Source: CAD feature listing. Evaluate the final solid. Frame: model axes, mm. A direction names the side the tool comes from. Give positions to 0.01 mm unless a question says otherwise; leave off trailing zeros. Write each loop counter-clockwise with the first axis right and the second up, starting at its lowest first coordinate (ties: lowest second). Pieces come first, ordered by that corner, then holes. Notation, with made-up numbers: (-35, -30) -> (-8, -30) arc R11 ccw to (-8, -19) -> close; hole circle Ø7 at (-35.5, -18.5). An arc over 180 degrees is marked (long way). Write item = value, one per line.
from build123d import *

# Parameters (mm, degrees)
CROQUIS1_W                   = 60
CROQUIS1_H                   = 60
CROQUIS1_W_2                 = 48
CROQUIS1_H_2                 = 48
SALIENTE_EXTRUIR1_DEPTH      = 17.5
SALIENTE_EXTRUIR1_DEPTH_BACK = 17.5
CROQUIS2_R                   = 9
SALIENTE_EXTRUIR2_DEPTH      = 2
CROQUIS3_R                   = 9
SALIENTE_EXTRUIR3_DEPTH      = 2
CROQUIS4_R                   = 9
SALIENTE_EXTRUIR4_DEPTH      = 2
CROQUIS5_R                   = 5
SALIENTE_EXTRUIR5_DEPTH      = 63
SALIENTE_EXTRUIR5_DEPTH_BACK = 63
CROQUIS6_R                   = 5
SALIENTE_EXTRUIR6_DEPTH      = 68
CUT_EXTRUDE1_REACH           = 62
SKETCH1_R                    = 1.6


with BuildPart() as part:
    # Croquis1 → Saliente-Extruir1 (new body, two sides)
    with BuildSketch(Plane(origin=(0, 0, 0), x_dir=(1, 0, 0), z_dir=(0, 1, 0))) as saliente_extruir1_sk:
        Rectangle(CROQUIS1_W, CROQUIS1_H)
        Rectangle(CROQUIS1_W_2, CROQUIS1_H_2, mode=Mode.SUBTRACT)
    extrude(amount=SALIENTE_EXTRUIR1_DEPTH)
    extrude(saliente_extruir1_sk.sketch, amount=-SALIENTE_EXTRUIR1_DEPTH_BACK)

    # Croquis2 → Saliente-Extruir2 (add)
    with BuildSketch(Plane.XY.offset(30)):
        Circle(CROQUIS2_R)
    extrude(amount=SALIENTE_EXTRUIR2_DEPTH)

    # Croquis3 → Saliente-Extruir3 (add)
    with BuildSketch(Plane(origin=(30, 0, 0), x_dir=(0, 0, -1), z_dir=(1, 0, 0))):
        Circle(CROQUIS3_R)
    extrude(amount=SALIENTE_EXTRUIR3_DEPTH)

    # Croquis4 → Saliente-Extruir4 (add)
    with BuildSketch(Plane.ZY.offset(30)):
        Circle(CROQUIS4_R)
    extrude(amount=SALIENTE_EXTRUIR4_DEPTH)

    # Croquis5 → Saliente-Extruir5 (add, two sides)
    with BuildSketch(Plane(origin=(0, 0, 0), x_dir=(0, 0, -1), z_dir=(1, 0, 0))) as saliente_extruir5_sk:
        Circle(CROQUIS5_R)
    extrude(amount=SALIENTE_EXTRUIR5_DEPTH)
    extrude(saliente_extruir5_sk.sketch, amount=-SALIENTE_EXTRUIR5_DEPTH_BACK)

    # Croquis6 → Saliente-Extruir6 (add)
    with BuildSketch(Plane.XY):
        Circle(CROQUIS6_R)
    extrude(amount=SALIENTE_EXTRUIR6_DEPTH)

    # Sketch1 → Cut-Extrude1 (cut, up to next)
    with BuildSketch(Plane.XY.offset(30), mode=Mode.PRIVATE) as cut_extrude1_sk1:
        with Locations((-20, 0)):
            Circle(SKETCH1_R)
    cut_extrude1_tool1 = extrude(cut_extrude1_sk1.sketch, amount=-CUT_EXTRUDE1_REACH, mode=Mode.PRIVATE) & part.part
    add(cut_extrude1_tool1.solids().sort_by_distance((-20, 0, 30))[0], mode=Mode.SUBTRACT)
    # Sketch1 → Cut-Extrude1 (cut, up to next)
    with BuildSketch(Plane.XY.offset(30), mode=Mode.PRIVATE) as cut_extrude1_sk2:
        with Locations((20, 0)):
            Circle(SKETCH1_R)
    cut_extrude1_tool2 = extrude(cut_extrude1_sk2.sketch, amount=-CUT_EXTRUDE1_REACH, mode=Mode.PRIVATE) & part.part
    add(cut_extrude1_tool2.solids().sort_by_distance((20, 0, 30))[0], mode=Mode.SUBTRACT)


solid = part.part
1) Material intervals for L1, parallel to Y at x = -20, z = 26.05; L2, parallel to Z at x = -9, y = -9; L3, parallel to Z at x = 6, y = -6, sorted ascending.
Computed:
L1 = -17.5 to -1.6, 1.6 to 17.5
L2 = -30 to -24, 24 to 30
L3 = -30 to -24, 24 to 32
2) Contact query for flat-ended pins moving along their axis: pin 1 (2.5 mm diameter, centred on x = 20, y = 0, fed in from +Z); pin 2 (6 mm diameter, centred on y = 4, z = 22.5, fed in from +X); pin 3 (1 mm diameter, centred on y = -2.5, z = -7, fed in from +X). Output: stop coordinate, or through.
Computed:
pin_1 = 5
pin_2 = 30
pin_3 = 32
3) Cut plane A-A (x = 14). Return the cut outline in (y, z).
Computed:
outline = (-17.5, -30) -> (17.5, -30) -> (17.5, -24) -> (-17.5, -24) -> close; (-17.5, 24) -> (17.5, 24) -> (17.5, 30) -> (-17.5, 30) -> close; circle Ø10 at (0, 0)
4) Cut plane C-C (y = 13.5). Return the cut outline in (x, z), then the cut area to 3 significant figures.
Computed:
outline = (-30, -30) -> (30, -30) -> (30, 30) -> (-30, 30) -> close; hole (-24, -24) -> (24, -24) -> (24, 24) -> (-24, 24) -> close
area = 1,300 mm²
5) Access query for faces 5 (the cylindrical face through (-47.28, -4.88, 1.08)), 6 (the cylindrical face through (-21.18, 1.08, 27.04)), 7 (the cylindrical face through (30.986, 8.923, 1.172)). Directions: +Z, -Z, +X, -X, +Y, -Y. A direction counts if a zero-diameter tool reaches every point of the face in a straight line with its end or side. Return the directions, or none.
Computed:
face_5 = -X
face_6 = +Z
face_7 = +X
6) Cut plane B-B (x = 0). Return the cut outline in (y, z).
Computed:
outline = (-17.5, -30) -> (17.5, -30) -> (17.5, -24) -> (-17.5, -24) -> close; (-17.5, 24) -> (-5, 24) -> (-5, 0) arc R5 ccw to (5, 0) -> (5, 24) -> (17.5, 24) -> (17.5, 30) -> (9, 30) -> (9, 32) -> (5, 32) -> (5, 68) -> (-5, 68) -> (-5, 32) -> (-9, 32) -> (-9, 30) -> (-17.5, 30) -> close
7) Cut plane D-D (z = 44). Return the cut outline in (x, y).
Computed:
outline = circle Ø10 at (0, 0)
8) Draft query along Z for faces 1 (the flat face through (-24, 0, 6)), 2 (the cylindrical face through (47.28, -4.88, 1.08)), 3 (the flat face through (-32, -4, 4)), 4 (the cylindrical face through (-4, 3, 14)). Return one class per face: pulls with the +Z half, pulls with the -Z half, needs draft (parallel to the pull), parting line crosses it, or undercut.
Computed:
face_1 = undercut
face_2 = parting line crosses it
face_3 = needs draft
face_4 = undercut
